```python
from build123d import *

# Parameters (mm, degrees)
SKETCH029_R     = 16
SKETCH029_R_2   = 10
SKETCH029_R_3   = 1.7
PAD008_DEPTH    = 7
PAD009_DEPTH    = 15
SKETCH031_R     = 1.8
POCKET020_DEPTH = 30
SKETCH032_W     = 46
SKETCH032_H     = 21.675207
PAD010_DEPTH    = 5


with BuildPart() as part:
    # Sketch029 → Pad008 (new body)
    with BuildSketch(Plane.XY):
        Circle(SKETCH029_R)
        Circle(SKETCH029_R_2, mode=Mode.SUBTRACT)
        with Locations((0, 12)):
            Circle(SKETCH029_R_3, mode=Mode.SUBTRACT)
        with Locations((-10.392305, -6)):
            Circle(SKETCH029_R_3, mode=Mode.SUBTRACT)
        with Locations((10.392305, -6)):
            Circle(SKETCH029_R_3, mode=Mode.SUBTRACT)
    extrude(amount=PAD008_DEPTH)

    # Sketch030 (on Face7 of Pad008) → Pad009 (join)
    with BuildSketch(Plane.XY.offset(7)):
        with BuildLine():
            ThreePointArc((-12.5, 16), (-28.5, 0), (-12.5, -16))
            Line((-12.5, -16), (12.5, -16))
            ThreePointArc((12.5, -16), (28.5, 0), (12.5, 16))
            Line((-12.5, 16), (12.5, 16))
        make_face()
    extrude(amount=PAD009_DEPTH)

    # Sketch031 (on Face17 of Pad009) → Pocket020 (cut)
    with BuildSketch(Plane.XY.offset(22)):
        with Locations((-17.491838, 7.554306)):
            Circle(SKETCH031_R)
        with Locations((-17.491838, -7.554306)):
            Circle(SKETCH031_R)
        with Locations((17.491838, -7.554306)):
            Circle(SKETCH031_R)
        with Locations((17.491838, 7.554306)):
            Circle(SKETCH031_R)
    extrude(amount=-POCKET020_DEPTH, mode=Mode.SUBTRACT)

    # Sketch032 (on Face9 of Pocket020) → Pad010 (join)
    with BuildSketch(Plane(origin=(0, 16, 0), x_dir=(-1, 0, 0), z_dir=(0, 1, 0))):
        with Locations((0, 10.914934)):
            Rectangle(SKETCH032_W, SKETCH032_H)
        with BuildLine():
            ThreePointArc((-16.6, 16), (-17, 16.4), (-17.4, 16))
            Line((-17.4, 16), (-17.4, 4))
            ThreePointArc((-17.4, 4), (-17, 3.6), (-16.6, 4))
            Line((-16.6, 16), (-16.6, 4))
        make_face(mode=Mode.SUBTRACT)
        with BuildLine():
            ThreePointArc((17.4, 16), (17, 16.4), (16.6, 16))
            Line((16.6, 16), (16.6, 4))
            ThreePointArc((16.6, 4), (17, 3.6), (17.4, 4))
            Line((17.4, 16), (17.4, 4))
        make_face(mode=Mode.SUBTRACT)
    extrude(amount=PAD010_DEPTH)


solid = part.part
```
Part model, mm, in its own coordinate system. A direction names the side the tool comes from. Give positions to 0.01 mm unless a question says otherwise; leave off trailing zeros. Loops run counter-clockwise (first coordinate to the right, second up) from the corner with the lowest first, then second, coordinate; pieces in that order, holes last. Notation, with made-up numbers: M -32.5,-31 L -26.5,-31 A15 cw -26.5,-5 Z; hole C 17.25,83 d2. An arc over 180 degrees is marked long. Return JSON: item names as keys, results as strings.
1) 3-axis set-ups, long thin cutter, end or side, ignore diameter. For faces 1 (the face through (17.4, 18, 10)), 2 (the face through (0, 12, 7)), 3 (the face through (0, 18, 0.077)), 4 (the face through (20, 0, 7)), 5 (the face through (-23, 18, 11)): which of +Z, -Z, +X, -X, +Y, -Y reach the whole face in a straight line?
Calculated:
{"face 1": "+Y", "face 2": "-Z", "face 3": "-Z, +X, -X, +Y", "face 4": "-Z, +X", "face 5": "+Z, -Z, -X, +Y"}
2) Drill centre lines: line 1 (X direction, y = 17, z = 11); line 2 (Y direction, x = 3, z = 4.5); line 3 (Z direction, x = 23.5, y = -6.5). Where is each one in solid material? Low to high.
Calculated:
{"line 1": "x = -23 to -17.4, -16.6 to 16.6, 17.4 to 23", "line 2": "y = -15.72 to -9.54, 9.54 to 15.72, 16 to 21", "line 3": "z = 7 to 22"}
3) Saw through at B-B, the plane y = 8.5. List the corners of the cut face in (x, z), then the cut area to 3 significant figures.
Calculated:
{"outline": "M -26.06,7 L -19.02,7 L -19.02,22 L -26.06,22 Z; M -15.96,7 L -13.56,7 L -13.56,0 L -5.27,0 L -5.27,7 L 5.27,7 L 5.27,0 L 13.56,0 L 13.56,7 L 15.96,7 L 15.96,22 L -15.96,22 Z; M 19.02,7 L 26.06,7 L 26.06,22 L 19.02,22 Z", "area": "806 mm2"}
4) Saw through at C-C, the plane x = 18. List the corners of the cut face in (y, z).
Calculated:
{"outline": "M -15.02,7 L -9.28,7 L -9.28,22 L -15.02,22 Z; M -5.83,7 L 5.83,7 L 5.83,22 L -5.83,22 Z; M 9.28,7 L 15.02,7 L 15.02,22 L 9.28,22 Z; M 16,0.08 L 21,0.08 L 21,21.75 L 16,21.75 Z"}
5) Pull direction X, two halves, no side cores. Call faces 6 (the face through (23, 18, 11)), 7 (the face through (0, 0, 22)), 8 (the face through (11.963, -6.651, 3.451)): released by +X, released by -X, zero draft, split by the parting line, or undercut.
Calculated:
{"face 6": "released by +X", "face 7": "zero draft", "face 8": "undercut"}
6) Saw through at D-D, the plane z = 19.5. List the corners of the cut face in (x, y).
Calculated:
{"outline": "M -23,16 L -12.5,16 A16 ccw -12.5,-16 L 12.5,-16 A16 ccw 12.5,16 L 23,16 L 23,21 L -23,21 Z; hole C -17.49,-7.55 d3.6; hole C -17.49,7.55 d3.6; hole C 17.49,-7.55 d3.6; hole C 17.49,7.55 d3.6"}
7) Flat gauge pins, fed straight in: pin 1 Ø1.5 at (y, z) = (18, 9.5) entering from +X; pin 2 Ø2 at (y, z) = (-10.5, 9.5) entering from +X; pin 3 Ø4 at (x, z) = (19.5, 9.5) entering from -Y; pin 4 Ø5 at (x, y) = (11, 7.5) entering from -Z. Where does each tip first touch, or does it go through?
Calculated:
{"pin 1": "stops at x = 23", "pin 2": "stops at x = 25.37", "pin 3": "stops at y = -15.2", "pin 4": "stops at z = 0"}
